Check sheet for the drawn part. Datum: minimum x, y, z corner. Units: mm. Coordinates: 2 decimals unless noted, no trailing zeros. Loops run counter-clockwise (first coordinate to the right, second up) from the corner with the lowest first, then second, coordinate; pieces in that order, holes last. Notation, with made-up numbers: M 48.25,34 L 88.25,34 A18 ccw 88.25,46 Z; hole C -13,62.5 d10. An arc over 180 degrees is marked long. Answer in a Markdown table with one row per item. Add a question column.
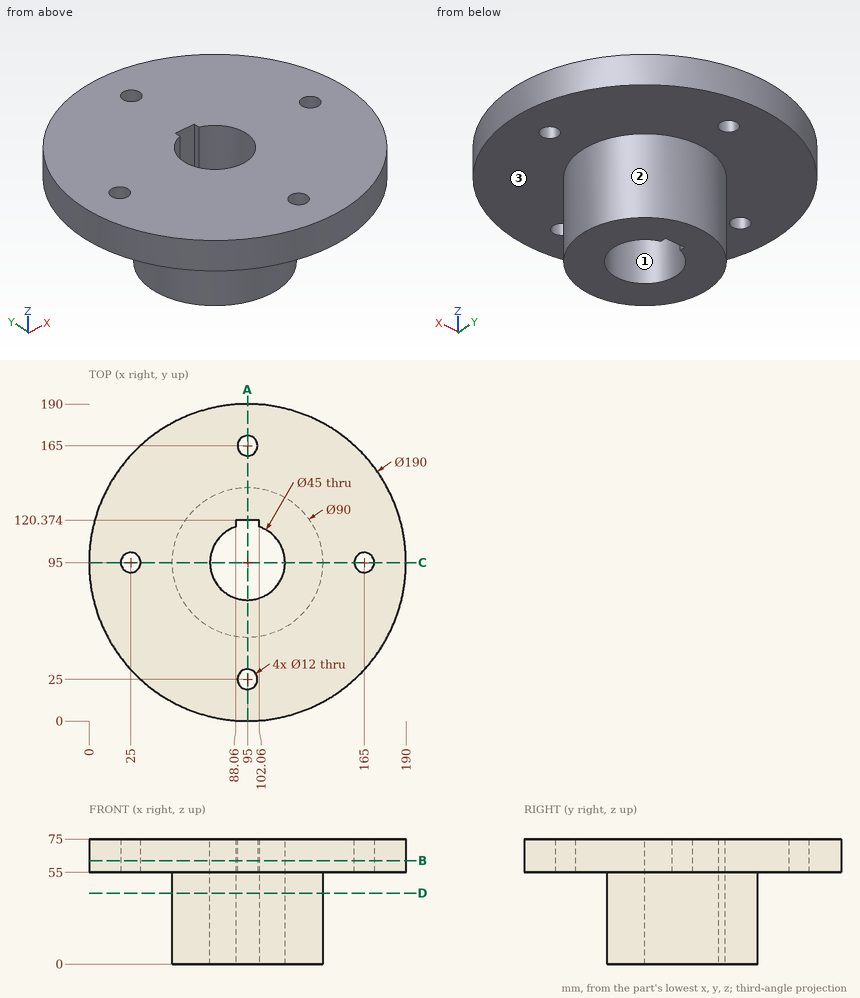
Q1. Mould release check, pull along Y, two halves, no side actions. Record for the marked faces 1, 2 and 3: released by +Y, released by -Y, zero draft, split by the parting line, or undercut.
Q2. Go/stop test with flat-tipped pins: pin 1 (3 mm diameter, centred on x = 123.5, z = 57.5, fed in from +Y); pin 2 (14 mm diameter, centred on x = 165, y = 95, fed in from -Z); pin 3 (2 mm diameter, centred on y = 118, z = 50.5, fed in from +X) (1 decimal); pin 4 (9.5 mm diameter, centred on x = 95, y = 165, fed in from -Z). Record where each tip stops, or that it passes through.
Q3. Cross-section at B-B (z = 62). Record the cut outline in (x, y).
Q4. Cross-section at C-C (y = 95). Record the cut outline in (x, z), plus the area to 4 significant figures.
Q5. Cross-section at D-D (z = 42.5). Record the cut outline in (x, y), plus the area to 3 significant figures.
Q6. Thickness scan on L1, parallel to Y at x = 95, z = 61.75; L2, parallel to Z at x = 78, y = 39; L3, parallel to Y at x = 95, z = 49. Record the ranges inside material, lowest first.
Q7. Cross-section at A-A (x = 95). Record the cut outline in (y, z), plus the area to 3 significant figures.
Answer key:
| question | item | result |
|---|---|---|
| 1 | face 1 | undercut |
| 1 | face 2 | split by the parting line |
| 1 | face 3 | zero draft |
| 2 | pin 1 | y = 186.08 |
| 2 | pin 2 | z = 55 |
| 2 | pin 3 | x = 134.3 |
| 2 | pin 4 | through |
| 3 | outline | C 95,95 d190; hole C 25,95 d12; hole M 88.06,116.4 A22.5 ccw long 102.06,116.36 L 102.06,120.37 L 88.06,120.37 Z; hole C 95,25 d12; hole C 95,165 d12; hole C 165,95 d12 |
| 4 | outline | M 0,55 L 19,55 L 19,75 L 0,75 Z; M 31,55 L 50,55 L 50,0 L 72.5,0 L 72.5,75 L 31,75 Z; M 117.5,0 L 140,0 L 140,55 L 159,55 L 159,75 L 117.5,75 Z; M 171,55 L 190,55 L 190,75 L 171,75 Z |
| 4 | area | 4,895 mm^2 |
| 5 | outline | C 95,95 d90; hole M 88.06,116.4 A22.5 ccw long 102.06,116.36 L 102.06,120.37 L 88.06,120.37 Z |
| 5 | area | 4,730 mm^2 |
| 6 | L1 | 0 to 19, 31 to 72.5, 120.37 to 159, 171 to 190 |
| 6 | L2 | 55 to 75 |
| 6 | L3 | 50 to 72.5, 120.37 to 140 |
| 7 | outline | M 0,55 L 19,55 L 19,75 L 0,75 Z; M 31,55 L 50,55 L 50,0 L 72.5,0 L 72.5,75 L 31,75 Z; M 120.37,0 L 140,0 L 140,55 L 159,55 L 159,75 L 120.37,75 Z; M 171,55 L 190,55 L 190,75 L 171,75 Z |
| 7 | area | 4,680 mm^2 |
